Design review of the part built by this model. Coordinates are the model's own, in mm. Face numbers are marked on the shaded views. A direction names the side the tool comes from. Round coordinates to 2 decimals unless told otherwise and drop trailing zeros. Order: outer loops, then holes, each group sorted by start corner. A loop starts at its lowest first (then second) coordinate and runs counter-clockwise, first axis right, second up.
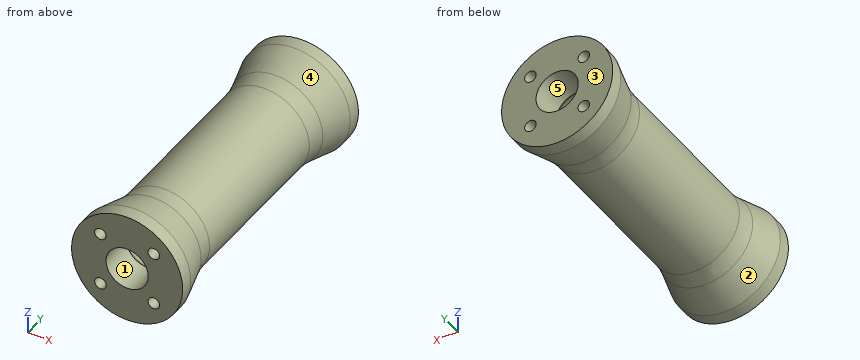
from build123d import *

# Parameters (mm, degrees)
SKETCH2_R          = 1.3
CUT_EXTRUDE1_DEPTH = 7
SKETCH5_R          = 4.75
CUT_EXTRUDE2_DEPTH = 68.360967927
FILLET1_R          = 15
FILLET2_R          = 4


with BuildPart() as part:
    # Sketch1 → Revolve1 (revolve)
    with BuildSketch(Plane.XY, mode=Mode.PRIVATE) as revolve1_sk:
        Polygon((0, -32.5), (0, 32.5), (-12.5, 32.5), (-12.5, 29.5), (-10, 20.5), (-10, -20.5), (-12.5, -29.5), (-12.5, -32.5), align=None)
    revolve(revolve1_sk.sketch.rotate(Axis((0, -32.5, 0), (0, 1, 0)), 270), axis=Axis((0, -32.5, 0), (0, 1, 0)))

    # Sketch2 → Cut-Extrude1 (cut)
    with BuildSketch(Plane(origin=(0, 32.5, 0), x_dir=(1, 0, 0), z_dir=(0, 1, 0))):
        with Locations(Location((-6, 6, 0), (0, 0, 270))):
            Circle(SKETCH2_R)
        with Locations(Location((6, 6, 0), (0, 0, 270))):
            Circle(SKETCH2_R)
        with Locations(Location((-6, -6, 0), (0, 0, 270))):
            Circle(SKETCH2_R)
        with Locations(Location((6, -6, 0), (0, 0, 270))):
            Circle(SKETCH2_R)
    cut_extrude1 = extrude(amount=-CUT_EXTRUDE1_DEPTH, mode=Mode.SUBTRACT)

    # Mirror1: Cut-Extrude1 across plane
    add(cut_extrude1.mirror(Plane.ZX), mode=Mode.SUBTRACT)

    # Sketch4 → Cut-Revolve1 (revolve, cut)
    with BuildSketch(Plane.XY):
        Polygon((0, 29.7), (-9, 20.7), (-9, -20.7), (0, -29.7), align=None)
    revolve(axis=Axis((0, 29.7, 0), (0, -1, 0)), mode=Mode.SUBTRACT)

    # Sketch5 → Cut-Extrude2 (cut, through all)
    with BuildSketch(Plane(origin=(0, 32.5, 0), x_dir=(1, 0, 0), z_dir=(0, 1, 0))):
        with Locations(Location((0, 0, 0), (0, 0, 270))):
            Circle(SKETCH5_R)
    extrude(amount=-CUT_EXTRUDE2_DEPTH, mode=Mode.SUBTRACT)

    # Fillet1
    fillet1_edges = [part.edges().sort_by_distance(p)[0] for p in [
        (0, -20.5, 10),
        (0, 20.5, 10),
    ]]
    fillet(fillet1_edges, radius=FILLET1_R)

    # Fillet2
    fillet2_edges = [part.edges().sort_by_distance(p)[0] for p in [
        (9, -20.7, 0),
        (9, 20.7, 0),
    ]]
    fillet(fillet2_edges, radius=FILLET2_R)


solid = part.part
1) The part is to be moulded in two halves that separate along X. For the marked faces 3, 4 and 5, say which applies: released by +X, released by -X, zero draft, split by the parting line, or undercut.
Results:
face 3: zero draft
face 4: split by the parting line
face 5: undercut
2) For the marked faces 1 and 2, list the 3-axis set-ups (+Z, -Z, +X, -X, +Y, -Y) from which the entire face can be reached by the end or side of a thin tool; tool diameter is ignored.
Results:
face 1: +Y, -Y
face 2: none
3) Take a section at A-A on y = 10.5. Give the boundary of the cut face in (x, z).
Results:
outline: circle Ø20 at (0, 0); hole circle Ø18 at (0, 0)
4) To check wall thickness, follow line 1 along X through (y, z) = (-30.25, 0); line 2 along X through (y, z) = (30.5, 6); line 3 along X through (y, z) = (-28.5, -6). State the ranges of each line that lie inside material, in increasing order.
Results:
line 1: x = -12.5 to -4.75, 4.75 to 12.5
line 2: x = -10.97 to -7.3, -4.7 to 4.7, 7.3 to 10.97
line 3: x = -10.65 to -7.3, -4.7 to 4.7, 7.3 to 10.65
5) Clearance check with flat-ended pins moving along their axes: P1, Ø1.3, axis at x = 6, z = -6.5, coming from the -Y side; P2, Ø1, axis at y = -25, z = 4, coming from the -X side; P3, Ø1.3, axis at x = -5.5, z = -6, coming from the +Y side. State where each tip first meets the part, or that it passes through.
Results:
P1: stops at y = -25.5
P2: stops at x = -10.75
P3: stops at y = 25.5
